The listing builds one solid part. Answer for the finished solid, in the listing's coordinates (mm). Face numbers are marked on the shaded views. A direction names the side the tool comes from. Coordinates: 2 decimals unless noted, no trailing zeros. Order: outer loops, then holes, each group sorted by start corner. A loop starts at its lowest first (then second) coordinate and runs counter-clockwise, first axis right, second up.
```python
from build123d import *

# Parameters (mm, degrees)
BOSS_EXTRUDE1_DEPTH   = 1
FILLET2_R             = 4
SKETCH2_W             = 20.4
SKETCH2_H             = 0.8
BOSS_EXTRUDE2_DEPTH   = 12.25
SKETCH3_W             = 0.8
SKETCH3_H             = 40
BOSS_EXTRUDE3_DEPTH   = 12.25
SKETCH5_W             = 0.8
SKETCH5_H             = 16.15
SKETCH5_H_2           = 10.15
BOSS_EXTRUDE4_DEPTH   = 12.25
FILLET3_R             = 1
SKETCH6_W             = 0.8
SKETCH6_H             = 10.15
BOSS_EXTRUDE5_DEPTH   = 0.6
SKETCH7_W             = 0.6
SKETCH7_H             = 10.15
EXTRUDE_THIN1_DEPTH   = 0.2
FILLET4_R             = 0.4
F_3_0MM_DOWEL_HOLE2_D = 3


with BuildPart() as part:
    # Sketch1 → Boss-Extrude1 (new body)
    with BuildSketch(Plane(origin=(-75.536427928, 0, 0), x_dir=(0, 0, -1), z_dir=(1, 0, 0))):
        Polygon((-25.5, 40.4), (-25.5, 54.4), (-14.2, 54.4), (-14.2, 78.4), (-10.2, 78.4), (-10.2, 54.4), (-10.2, 40.4), (10.2, 40.4), (10.2, 54.4), (10.2, 78.4), (14.2, 78.4), (14.2, 54.4), (25.5, 54.4), (25.5, 40.4), (25.5, 34.4), (-25.5, 34.4), align=None)
    extrude(amount=BOSS_EXTRUDE1_DEPTH)

    # Fillet2
    fillet2_edges = [part.edges().sort_by_distance(p)[0] for p in [
        (-75.036427928, 54.4, -25.5),
        (-75.036427928, 34.4, -25.5),
        (-75.036427928, 34.4, 25.5),
        (-75.036427928, 54.4, 25.5),
    ]]
    fillet(fillet2_edges, radius=FILLET2_R)

    # Sketch2 → Boss-Extrude2 (add)
    with BuildSketch(Plane(origin=(-74.536427928, 0, 0), x_dir=(0, 0, -1), z_dir=(1, 0, 0))):
        with Locations((0, 38.8)):
            Rectangle(SKETCH2_W, SKETCH2_H)
    extrude(amount=BOSS_EXTRUDE2_DEPTH)

    # Sketch3 → Boss-Extrude3 (add)
    with BuildSketch(Plane(origin=(-74.536427928, 0, 0), x_dir=(0, 0, -1), z_dir=(1, 0, 0))):
        with Locations((-10.6, 58.4)):
            Rectangle(SKETCH3_W, SKETCH3_H)
    extrude(amount=BOSS_EXTRUDE3_DEPTH)

    # Sketch5 → Boss-Extrude4 (add)
    with BuildSketch(Plane(origin=(-74.536427928, 0, 0), x_dir=(0, 0, -1), z_dir=(1, 0, 0))):
        with Locations((10.6, 46.475)):
            Rectangle(SKETCH5_W, SKETCH5_H)
        with Locations((10.6, 73.325)):
            Rectangle(SKETCH5_W, SKETCH5_H_2)
    extrude(amount=BOSS_EXTRUDE4_DEPTH)

    # Fillet3
    fillet3_edges = [part.edges().sort_by_distance(p)[0] for p in [
        (-74.536427928, 46.475, -11),
        (-74.536427928, 73.325, -11),
        (-74.536427928, 38.4, 0),
        (-74.536427928, 58.4, 11),
    ]]
    fillet(fillet3_edges, radius=FILLET3_R)

    # Sketch6 → Boss-Extrude5 (add)
    with BuildSketch(Plane(origin=(-62.286427928, 0, 0), x_dir=(0, 0, -1), z_dir=(1, 0, 0))):
        Polygon((-11, 38.4), (11, 38.4), (11, 54.55), (10.2, 54.55), (10.2, 39.2), (-10.2, 39.2), (-10.2, 78.4), (-11, 78.4), align=None)
        with Locations((10.6, 73.325)):
            Rectangle(SKETCH6_W, SKETCH6_H)
    extrude(amount=BOSS_EXTRUDE5_DEPTH)

    # Sketch7 → Extrude-Thin1 (add)
    with BuildSketch(Plane(origin=(-61.686427928, 0, 0), x_dir=(0, 0, -1), z_dir=(1, 0, 0))):
        with Locations((9.9, 73.325)):
            Rectangle(SKETCH7_W, SKETCH7_H)
        Polygon((10.2, 54.55), (10.2, 39.2), (-10.2, 39.2), (-10.2, 78.4), (-9.6, 78.4), (-9.6, 39.8), (9.6, 39.8), (9.6, 54.55), align=None)
    extrude(amount=-EXTRUDE_THIN1_DEPTH)

    # Fillet4
    fillet4_edges = [part.edges().sort_by_distance(p)[0] for p in [
        (-61.886427928, 73.325, -10.2),
        (-61.886427928, 46.875, -10.2),
        (-61.886427928, 39.2, 0),
        (-61.886427928, 58.8, 10.2),
    ]]
    fillet(fillet4_edges, radius=FILLET4_R)

    # Ø3.0mm Dowel Hole2 (through all)
    with Locations(Plane(origin=(-74.536427928, 0, 0), x_dir=(0, 0, -1), z_dir=(1, 0, 0))):
        with Locations((21.5, 47.4), (-21.5, 47.4)):
            Hole(F_3_0MM_DOWEL_HOLE2_D / 2)


solid = part.part
```
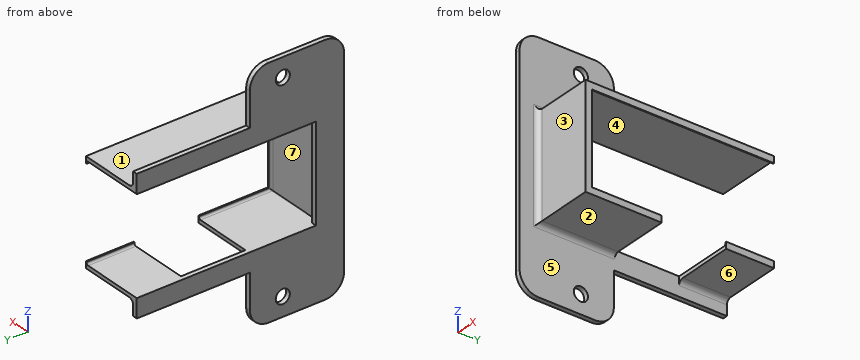
(1) Find section D-D (y = 56). Write down the section's boundary in (x, z), and give its area (3 significant figures).
(2) For the marked faces 1, 2 and 3, determine the directions among +Z, -Z, +X, -X, +Y, -Y from which every point of the face is accessible in a straight line to the end or side of a thin tool.
(3) Consider line 1 (Y direction, x = -74.8, z = -21.5); line 2 (Z direction, x = -70, y = 74); line 3 (Y direction, x = -71.75, z = 8). Determine where each line is inside the solid, lowest interval first.
(4) Find section C-C (y = 47.4). Write down the section's boundary in (x, z).
(5) Find section B-B (x = -69). Write down the section's boundary in (y, z).
(6) Find section A-A (y = 41.5). Write down the section's boundary in (x, z).
(7) The mould has two halves that part along Z. Classify the marked faces 4, 5, 6 and 7: released by +Z, released by -Z, zero draft, split by the parting line, or undercut.
(8) Each of these flat-tipped pins is pushed along its axis until it touches: pin 1 Ø6 at (x, y) = (-70, 65) entering from +Z; pin 2 Ø2.5 at (y, z) = (47.4, -21.5) entering from -X; pin 3 Ø0.5 at (x, y) = (-75, 64) entering from -Z; pin 4 Ø1.1 at (x, z) = (-75, 19.5) entering from +Y. Where does it stop, or does it pass through?
Findings below:
1. outline: (-75.54, -14.2) - (-74.54, -14.2) - (-74.54, -10.2) - (-75.54, -10.2) - close; (-75.54, 10.2) - (-62.29, 10.2) arc R0.4 cw to (-61.89, 9.8) - (-61.89, 9.6) - (-61.69, 9.6) - (-61.69, 11) - (-73.54, 11) arc R1 cw to (-74.54, 12) - (-74.54, 14.2) - (-75.54, 14.2) - close
1. area: 18.6 mm2
2. face 1: +Z, +X, +Y, -Y
2. face 2: -Z, +X, +Y, -Y
2. face 3: +Z, -Z, +X, -Y
3. line 1: y = 34.4 to 45.9, 48.9 to 54.4
3. line 2: z = -11 to -10.2, 10.2 to 11
3. line 3: y = 38.4 to 39.2
4. outline: (-75.54, -25.5) - (-74.54, -25.5) - (-74.54, -23) - (-75.54, -23) - close; (-75.54, -20) - (-74.54, -20) - (-74.54, -12) arc R1 cw to (-73.54, -11) - (-61.69, -11) - (-61.69, -9.6) - (-61.89, -9.6) - (-61.89, -9.8) arc R0.4 cw to (-62.29, -10.2) - (-75.54, -10.2) - close; (-75.54, 10.2) - (-62.29, 10.2) arc R0.4 cw to (-61.89, 9.8) - (-61.89, 9.6) - (-61.69, 9.6) - (-61.69, 11) - (-73.54, 11) arc R1 cw to (-74.54, 12) - (-74.54, 20) - (-75.54, 20) - close; (-75.54, 23) - (-74.54, 23) - (-74.54, 25.5) - (-75.54, 25.5) - close
5. outline: (38.4, -11) - (54.55, -11) - (54.55, -10.2) - (39.2, -10.2) - (39.2, 10.2) - (78.4, 10.2) - (78.4, 11) - (38.4, 11) - close; (68.25, -11) - (78.4, -11) - (78.4, -10.2) - (68.25, -10.2) - close
6. outline: (-75.54, -25.5) - (-74.54, -25.5) - (-74.54, -12) arc R1 cw to (-73.54, -11) - (-61.69, -11) - (-61.69, -9.6) - (-61.89, -9.6) - (-61.89, -9.8) arc R0.4 cw to (-62.29, -10.2) - (-75.54, -10.2) - close; (-75.54, 10.2) - (-62.29, 10.2) arc R0.4 cw to (-61.89, 9.8) - (-61.89, 9.6) - (-61.69, 9.6) - (-61.69, 11) - (-73.54, 11) arc R1 cw to (-74.54, 12) - (-74.54, 25.5) - (-75.54, 25.5) - close
7. face 4: undercut
7. face 5: zero draft
7. face 6: released by -Z
7. face 7: undercut
8. pin 1: stops at z = 11
8. pin 2: passes through
8. pin 3: stops at z = -14.2
8. pin 4: stops at y = 54.4
